from build123d import *

# Parameters (mm, degrees)
SKETCH1_R            = 10
BOSS_EXTRUDE1_DEPTH  = 130
SKETCH2_R            = 16
BOSS_EXTRUDE2_DEPTH  = 10
SKETCH3_R            = 10
BOSS_EXTRUDE4_DEPTH  = 5
SKETCH6_R            = 16
BOSS_EXTRUDE5_DEPTH  = 55
SKETCH7_R            = 17.5
BOSS_EXTRUDE6_DEPTH  = 20
SKETCH8_R            = 20
BOSS_EXTRUDE7_DEPTH  = 10
SKETCH9_R            = 18
BOSS_EXTRUDE8_DEPTH  = 10
SKETCH10_R           = 13
BOSS_EXTRUDE9_DEPTH  = 26
BOSS_EXTRUDE10_DEPTH = 8


with BuildPart() as part:
    # Sketch1 → Boss-Extrude1 (new body)
    with BuildSketch(Plane.XY):
        Circle(SKETCH1_R)
    extrude(amount=-BOSS_EXTRUDE1_DEPTH)

    # Sketch2 → Boss-Extrude2 (add)
    with BuildSketch(Plane(origin=(0, 0, -130), x_dir=(-1, 0, 0), z_dir=(0, 0, -1))):
        Circle(SKETCH2_R)
    extrude(amount=BOSS_EXTRUDE2_DEPTH)

    # Sketch3 → Boss-Extrude4 (add)
    with BuildSketch(Plane(origin=(0, 0, -140), x_dir=(-1, 0, 0), z_dir=(0, 0, -1))):
        Circle(SKETCH3_R)
    extrude(amount=BOSS_EXTRUDE4_DEPTH)

    # Sketch6 → Boss-Extrude5 (add)
    with BuildSketch(Plane(origin=(0, 0, -145), x_dir=(-1, 0, 0), z_dir=(0, 0, -1))):
        Circle(SKETCH6_R)
    extrude(amount=BOSS_EXTRUDE5_DEPTH)

    # Sketch7 → Boss-Extrude6 (add)
    with BuildSketch(Plane(origin=(0, 0, -200), x_dir=(-1, 0, 0), z_dir=(0, 0, -1))):
        Circle(SKETCH7_R)
    extrude(amount=BOSS_EXTRUDE6_DEPTH)

    # Sketch8 → Boss-Extrude7 (add)
    with BuildSketch(Plane(origin=(0, 0, -220), x_dir=(-1, 0, 0), z_dir=(0, 0, -1))):
        Circle(SKETCH8_R)
    extrude(amount=BOSS_EXTRUDE7_DEPTH)

    # Sketch9 → Boss-Extrude8 (add)
    with BuildSketch(Plane(origin=(0, 0, -230), x_dir=(-1, 0, 0), z_dir=(0, 0, -1))):
        with Locations((0, 20)):
            Circle(SKETCH9_R)
    extrude(amount=BOSS_EXTRUDE8_DEPTH)

    # Sketch10 → Boss-Extrude9 (add)
    with BuildSketch(Plane(origin=(0, 0, -240), x_dir=(-1, 0, 0), z_dir=(0, 0, -1))):
        with Locations((0, 20)):
            Circle(SKETCH10_R)
    extrude(amount=BOSS_EXTRUDE9_DEPTH)

    # Sketch11 → Boss-Extrude10 (add)
    with BuildSketch(Plane.XY.offset(-230)):
        with BuildLine():
            Line((-16.914467174, 26.15636258), (-25.189753073, 3.420201433))
            ThreePointArc((-25.189753073, 3.420201433), (-26.92623485, 0.41252677), (-29.586679281, -1.819851171))
            Line((-29.586679281, -1.819851171), (-62.4486633, -20.792726491))
            ThreePointArc((-62.4486633, -20.792726491), (-64.686631077, -23.525461465), (-64.560098939, -27.055380703))
            ThreePointArc((-64.560098939, -27.055380703), (0, -70), (64.560098939, -27.055380703))
            ThreePointArc((64.560098939, -27.055380703), (64.686631077, -23.525461465), (62.4486633, -20.792726491))
            Line((62.4486633, -20.792726491), (29.586679281, -1.819851171))
            ThreePointArc((29.586679281, -1.819851171), (26.92623485, 0.41252677), (25.189753073, 3.420201433))
            Line((25.189753073, 3.420201433), (16.914467174, 26.15636258))
            ThreePointArc((16.914467174, 26.15636258), (0, 2), (-16.914467174, 26.15636258))
        make_face()
    extrude(amount=-BOSS_EXTRUDE10_DEPTH)


solid = part.part
For this review, take the finished solid that the model builds, in its own axes (mm). A direction names the side the tool comes from. Coordinates: 2 decimals unless noted, no trailing zeros. Loops run counter-clockwise (first coordinate to the right, second up) from the corner with the lowest first, then second, coordinate; pieces in that order, holes last. Notation, with made-up numbers: (-2.75, 72.5) - (40.25, 72.5) arc R27 ccw to (40.25, 93.5) - close; hole circle Ø10 at (71, -8). An arc over 180 degrees is marked (long way). Use a Markdown table: item, result. Add a question column.
Item 1: We need section B-B (z = -82). Give the boundary of the cut face in (x, y), and give its area (3 significant figures).
Item 2: Mouldability with a two-part tool opening along Z and no side actions: class faces 1 (the face through (2.17, -9.76, -142.46)), 2 (the face through (3.47, -15.62, -172.12)), 3 (the face through (-7.7, -14.2, -200)) as pulls with the +Z half, pulls with the -Z half, needs draft (parallel to the pull), parting line crosses it, or undercut.
Item 3: For line 1 (Z direction, x = 4, y = -54.5); line 2 (Z direction, x = -2.5, y = 22.5); line 3 (Y direction, x = -3, z = -191.5), list the stretches that pass through material, from the lowest coordinate up.
Item 4: Insertion check: pin 1 Ø3 at (y, z) = (12, -175) entering from -X; pin 2 Ø5 at (x, z) = (18, -236.5) entering from +Y; pin 3 Ø8 at (x, y) = (-48, -17.5) entering from +Z; pin 4 Ø12 at (x, y) = (-2, 6.5) entering from +Z. Each pin has a flat end and moves straight along its axis. Give the tip position at first contact, or say it passes through.
Item 5: We need section C-C (y = -58.5). Give the boundary of the cut face in (x, z).
Item 6: Tool access review of faces 4 (the face through (2.343, 37.847, -236.041)), 5 (the face through (-2.17, -9.76, -64.09)), 6 (the face through (-26.895, 0.45, -233.944)), 7 (the face through (-10.4, 0.2, -145)): name each direction out of +Z, -Z, +X, -X, +Y, -Y from which nothing blocks a thin tool from reaching the whole face with its end or side.
Item 7: We need section D-D (x = 40.5). Give the boundary of the cut face in (y, z), and give its area (3 significant figures).
Results list:
| question | item | result |
|---|---|---|
| 1 | outline | circle Ø20 at (0, 0) |
| 1 | area | 314 mm^2 |
| 2 | face 1 | undercut |
| 2 | face 2 | needs draft |
| 2 | face 3 | pulls with the +Z half |
| 3 | line 1 | z = -238 to -230 |
| 3 | line 2 | z = -266 to -230 |
| 3 | line 3 | y = -15.72 to 15.72 |
| 4 | pin 1 | stops at x = -12.07 |
| 4 | pin 2 | stops at y = 29.15 |
| 4 | pin 3 | stops at z = -230 |
| 4 | pin 4 | stops at z = 0 |
| 5 | outline | (-38.44, -238) - (38.44, -238) - (38.44, -230) - (-38.44, -230) - close |
| 6 | face 4 | -Z |
| 6 | face 5 | +Z |
| 6 | face 6 | +Z, -Z, -X, +Y |
| 6 | face 7 | none |
| 7 | outline | (-57.09, -238) - (-8.12, -238) - (-8.12, -230) - (-57.09, -230) - close |
| 7 | area | 392 mm^2 |
